Source: CAD feature listing. Evaluate the final solid. Frame: model axes, mm. Face numbers are marked on the shaded views. A direction names the side the tool comes from. Round coordinates to 2 decimals unless told otherwise and drop trailing zeros. Order: outer loops, then holes, each group sorted by start corner. A loop starts at its lowest first (then second) coordinate and runs counter-clockwise, first axis right, second up. Notation, with made-up numbers: (52, -28.5) -> (59, -28.5) arc R21 ccw to (59, 9.5) -> close; hole circle Ø10 at (50, -3). An arc over 180 degrees is marked (long way). Answer as CSV lines item,"result".
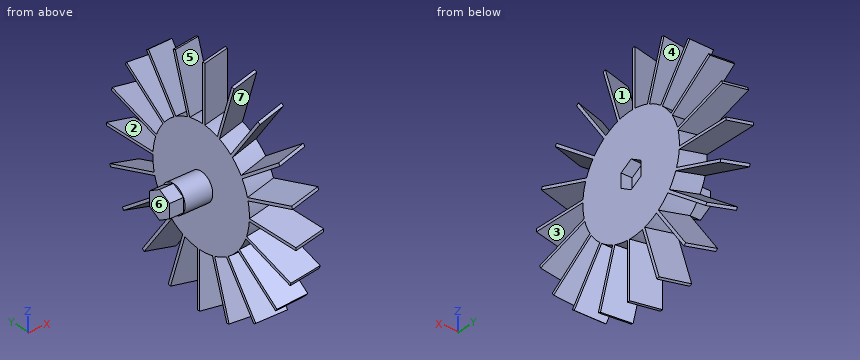
from build123d import *

# Parameters (mm, degrees)
SKETCH_R           = 10.375
PAD_DEPTH          = 5
POCKET_DEPTH       = 2
PAD001_DEPTH       = 10
PAD001_DEPTH_BACK  = 1
POLARPATTERN_COUNT = 20
SKETCH003_R        = 2.5
PAD002_DEPTH       = 5
PAD003_DEPTH       = 2.5


with BuildPart() as part:
    # Sketch → Pad (new body)
    with BuildSketch(Plane.YZ):
        Circle(SKETCH_R)
    extrude(amount=PAD_DEPTH)

    # Sketch001 (on Face3 of Pad) → Pocket (cut)
    with BuildSketch(Plane.YZ.offset(5)):
        Polygon((2.165064, 1.25), (0, 2.5), (-2.165064, 1.25), (-2.165064, -1.25), (0, -2.5), (2.165064, -1.25), align=None)
    extrude(amount=-POCKET_DEPTH, mode=Mode.SUBTRACT)

    # Sketch002 (on DatumPlane) → Pad001 (join, two sides)
    with BuildSketch(Plane.ZX.offset(10.375)) as pad001_sk:
        Polygon((0.8, 0), (-0.3, 5), (-0.8, 5), (0.3, 0), align=None)
    pad001 = extrude(amount=PAD001_DEPTH) + extrude(pad001_sk.sketch, amount=-PAD001_DEPTH_BACK)

    # PolarPattern: Pad001 ×20 about axis
    polarpattern_axis = Axis((0, 0, 0), (1, 0, 0))
    for i in range(1, POLARPATTERN_COUNT):
        add(pad001.rotate(polarpattern_axis, i * 360 / POLARPATTERN_COUNT))

    # Sketch003 (on Face2 of PolarPattern) → Pad002 (join)
    with BuildSketch(Plane(origin=(0, 0, 0), x_dir=(0, 1, 0), z_dir=(-1, 0, 0))):
        Circle(SKETCH003_R)
    extrude(amount=PAD002_DEPTH)

    # Sketch004 (on Face108 of Pad002) → Pad003 (join)
    with BuildSketch(Plane(origin=(-5, 0, 0), x_dir=(0, 1, 0), z_dir=(-1, 0, 0))):
        Polygon((2.165064, 1.25), (0, 2.5), (-2.165064, 1.25), (-2.165064, -1.25), (0, -2.5), (2.165064, -1.25), align=None)
    extrude(amount=PAD003_DEPTH)


solid = part.part
1. Line query: L1, parallel to Y at x = 2, z = 16; L2, parallel to Z at x = 1, y = 12; L3, parallel to Y at x = 1.5, z = 18. Output: solid intervals per line, ascending. Write a range as [from, to].
Results below:
L1,"[-12.07, -11.45], [-5.58, -5.05], [-0.36, 0.14], [4.82, 5.35], [11.18, 11.8]"
L2,"[-16.38, -15.53], [-8.62, -8], [-3.81, -3.29], [0.08, 0.58], [3.98, 4.51], [8.82, 9.44]"
L3,"[-6.34, -5.82], [-0.47, 0.03], [5.35, 5.88]"
2. Mould query, pull axis Z, two halves, no side actions, for the marked faces 5, 6 and 7. Classes: released by +Z, released by -Z, zero draft, split by the parting line, or undercut.
Results below:
face 5,"released by +Z"
face 6,"zero draft"
face 7,"undercut"
3. Section query A-A on z = 18.5. Return loops of the section in (x, y).
Results below:
outline,"(0, -6.85) -> (5, -5.7) -> (5, -5.17) -> (0, -6.33) -> close; (0, -0.8) -> (5, 0.3) -> (5, 0.8) -> (0, -0.3) -> close; (0, 5.17) -> (5, 6.33) -> (5, 6.85) -> (0, 5.7) -> close"
4. Reachability of the marked faces 1, 2, 3 and 4 from +Z, -Z, +X, -X, +Y, -Y: full face, straight path, thin tool, end or side. Return the list, or none.
Results below:
face 1,"+Z, -X"
face 2,"+X, +Y"
face 3,"+X, -Y"
face 4,"-X"
5. Pin query (flat end, axial travel): pin 1 (12 mm diameter, centred on y = -10, z = 3, fed in from -X); pin 2 (1.3 mm diameter, centred on y = -0.5, z = -0.5, fed in from +X); pin 3 (1.5 mm diameter, centred on x = 0.5, y = 15, fed in from +Z). Return the tip coordinate at first contact, or that it passes through.
Results below:
pin 1,"x = 0"
pin 2,"x = 3"
pin 3,"z = 12.33"
